```python
from build123d import *

# Parameters (mm, degrees)
SKETCH1_W           = 235
SKETCH1_H           = 235
BOSS_EXTRUDE1_DEPTH = 1
SKETCH2_R           = 1.5
BOSS_EXTRUDE2_DEPTH = 1
FILLET1_R           = 5
CHAMFER1_SIZE       = 15


with BuildPart() as part:
    # Sketch1 → Boss-Extrude1 (new body)
    with BuildSketch(Plane(origin=(0, 0, 0), x_dir=(1, 0, 0), z_dir=(0, 1, 0))):
        Rectangle(SKETCH1_W, SKETCH1_H)
    extrude(amount=BOSS_EXTRUDE1_DEPTH)

    # Sketch2 → Boss-Extrude2 (add)
    with BuildSketch(Plane(origin=(0, 0, 0), x_dir=(1, 0, 0), z_dir=(0, 1, 0))):
        Polygon((-82.041451884, 117.5), (-78, 124.5), (-62, 124.5), (-57.958548116, 117.5), align=None)
        with Locations((-75, 121)):
            Circle(SKETCH2_R, mode=Mode.SUBTRACT)
        with Locations((-65, 121)):
            Circle(SKETCH2_R, mode=Mode.SUBTRACT)
        Polygon((57.958548116, 117.5), (82.041451884, 117.5), (78, 124.5), (62, 124.5), align=None)
        with Locations((65, 121)):
            Circle(SKETCH2_R, mode=Mode.SUBTRACT)
        with Locations((75, 121)):
            Circle(SKETCH2_R, mode=Mode.SUBTRACT)
    extrude(amount=BOSS_EXTRUDE2_DEPTH)

    # Fillet1
    fillet1_edges = [part.edges().sort_by_distance(p)[0] for p in [
        (-82.041451884, 0.5, -117.5),
        (-57.958548116, 0.5, -117.5),
        (-62, 0.5, -124.5),
        (-78, 0.5, -124.5),
        (62, 0.5, -124.5),
        (57.958548116, 0.5, -117.5),
        (82.041451884, 0.5, -117.5),
        (78, 0.5, -124.5),
    ]]
    fillet(fillet1_edges, radius=FILLET1_R)

    # Chamfer1
    chamfer1_edges = [part.edges().sort_by_distance(p)[0] for p in [
        (-117.5, 0.5, -117.5),
        (117.5, 0.5, -117.5),
        (117.5, 0.5, 117.5),
        (-117.5, 0.5, 117.5),
    ]]
    chamfer(chamfer1_edges, length=CHAMFER1_SIZE)


solid = part.part
```
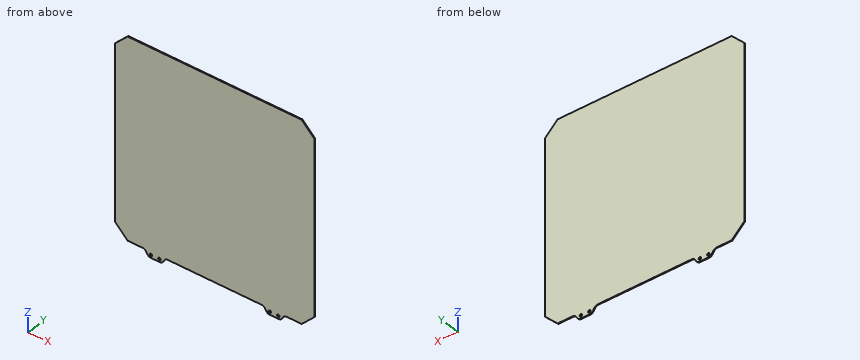
The listing builds one solid part. Answer for the finished solid, in the listing's coordinates (mm). Give positions to 0.01 mm unless a question says otherwise; leave off trailing zeros. Loops run counter-clockwise (first coordinate to the right, second up) from the corner with the lowest first, then second, coordinate; pieces in that order, holes last. Notation, with made-up numbers: (46.5, 83.25) - (86.5, 83.25) arc R30 cw to (86.5, 110.25) - close; hole circle Ø4 at (43.5, -25). An arc over 180 degrees is marked (long way). Return JSON: item names as keys, results as strings. Group by question number.
1. Straight lines are drawn through the part: line 1 (Z direction, x = 65, y = 0.3); line 2 (X direction, y = 0.5, z = -121); line 3 (Z direction, x = -95.5, y = 0.2). For each, find the intervals that lie inside material, in ascending order. Write a range as [from, to].
2. Find section B-B (x = 89). Write down the section's boundary in (y, z).
3. Find section A-A (y = 0.4). Write down the section's boundary in (x, z), then the cut area to 3 significant figures.
Verdict:
{
 "1": {"line 1": "z = [-124.5, -122.5], [-119.5, 117.5]", "line 2": "x = [-80.02, -76.5], [-73.5, -66.5], [-63.5, -59.98], [59.98, 63.5], [66.5, 73.5], [76.5, 80.02]", "line 3": "z = [-117.5, 117.5]"},
 "2": {"outline": "(0, -117.5) - (1, -117.5) - (1, 117.5) - (0, 117.5) - close"},
 "3": {"outline": "(-117.5, -102.5) - (-102.5, -117.5) - (-84.93, -117.5) arc R5 cw to (-80.6, -120) - (-79.44, -122) arc R5 ccw to (-75.11, -124.5) - (-64.89, -124.5) arc R5 ccw to (-60.56, -122) - (-59.4, -120) arc R5 cw to (-55.07, -117.5) - (55.07, -117.5) arc R5 cw to (59.4, -120) - (60.56, -122) arc R5 ccw to (64.89, -124.5) - (75.11, -124.5) arc R5 ccw to (79.44, -122) - (80.6, -120) arc R5 cw to (84.93, -117.5) - (102.5, -117.5) - (117.5, -102.5) - (117.5, 102.5) - (102.5, 117.5) - (-102.5, 117.5) - (-117.5, 102.5) - close; hole circle Ø3 at (-75, -121); hole circle Ø3 at (-65, -121); hole circle Ø3 at (65, -121); hole circle Ø3 at (75, -121)", "area": "55,000 mm^2"}
}
